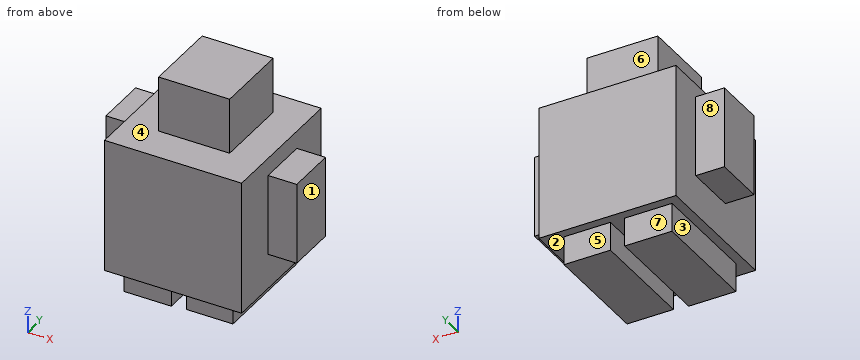
```python
from build123d import *

# Parameters (mm, degrees)
F0_W      = 74.0942507982
F0_H      = 74.6015533805
F1_DEPTH  = 72.4732205272
F2_W      = 38.3877456188
F2_H      = 40.8380180597
F3_DEPTH  = 30.0961155444
F4_W      = 26.9601941109
F4_H      = 43.9190119505
F5_DEPTH  = 15.5
F6_W      = 27.8298556805
F6_H      = 43.9190119505
F7_DEPTH  = 15.5
F8_W      = 25.5186259747
F8_H      = 59.9911510944
F9_DEPTH  = 15.5
F10_W     = 25.0709354877
F10_H     = 59.0957701206
F11_DEPTH = 15.5


with BuildPart() as f1:
    # F0 (on Top) → F1 (new body)
    with BuildSketch(Plane.XY):
        with Locations((-37.0471253991, 37.3007766902)):
            Rectangle(F0_W, F0_H)
    extrude(amount=F1_DEPTH)

    # F2 (on face) → F3 (join)
    with BuildSketch(Plane.XY.offset(72.4732205272)):
        with Locations((-36.9584262371, 40.0212556124)):
            Rectangle(F2_W, F2_H)
    extrude(amount=F3_DEPTH)

    # F4 (on face) → F5 (join)
    with BuildSketch(Plane.YZ):
        with Locations((38.2660329342, 40.9622490406)):
            Rectangle(F4_W, F4_H)
    extrude(amount=F5_DEPTH)

    # F6 (on face) → F7 (join)
    with BuildSketch(Plane(origin=(-74.0942507982, 0, 0), x_dir=(0, -1, 0), z_dir=(-1, 0, 0))):
        with Locations((-42.1796441078, 43.3538928628)):
            Rectangle(F6_W, F6_H)
    extrude(amount=F7_DEPTH)

    # F8 (on face) → F9 (join)
    with BuildSketch(Plane(origin=(0, 0, 0), x_dir=(1, 0, 0), z_dir=(0, 0, -1))):
        with Locations((-56.3197880983, -39.6210104227)):
            Rectangle(F8_W, F8_H)
    extrude(amount=F9_DEPTH)

    # F10 (on face) → F11 (join)
    with BuildSketch(Plane(origin=(0, 0, 0), x_dir=(1, 0, 0), z_dir=(0, 0, -1))):
        with Locations((-23.4141945839, -40.2925610542)):
            Rectangle(F10_W, F10_H)
    extrude(amount=F11_DEPTH)


solid = f1.part
```
The model under review builds one solid part; all positions refer to its coordinate system, in mm. Face numbers are marked on the shaded views. A direction names the side the tool comes from. Round coordinates to 2 decimals unless told otherwise and drop trailing zeros. Write each loop counter-clockwise with the first axis right and the second up, starting at its lowest first coordinate (ties: lowest second). Pieces come first, ordered by that corner, then holes. Notation, with made-up numbers: (85.25, 40.25) - (128.25, 40.25) arc R18 cw to (128.25, 56.25) - close; hole circle Ø5 at (-28, 44.25). An arc over 180 degrees is marked (long way). Answer as CSV lines item,"result". Start each with the question number.
(1) We need section D-D on x = -48. State the section outline as (y, z) points.
(2) Draft analysis for pull direction X (two halves, no side actions). For the marked faces 1, 2, 3 and 4, state which applies: pulls with the +X half, pulls with the -X half, needs draft (parallel to the pull), parting line crosses it, or undercut.
(3) To check wall thickness, follow line 1 (Y direction, x = -20.5, z = 96.5); line 2 (X direction, y = 60, z = 34.5); line 3 (Y direction, x = -77.5, z = 57). State the ranges of each line that lie inside material, in increasing order.
(4) We need section C-C on z = 61. State the section outline as (x, y) points.
(5) For the marked faces 5, 6, 7 and 8, list the 3-axis set-ups (+Z, -Z, +X, -X, +Y, -Y) from which the entire face can be reached by the end or side of a thin tool; tool diameter is ignored.
(6) We need section A-A on y = 42. State the section outline as (x, z) points.
(7) We need section B-B on x = -62.5. State the section outline as (y, z) points, plus the area to 3 significant figures.
(8) For pin 1 Ø12.5 at (x, z) = (-51.5, -4) entering from +Y; pin 2 Ø8 at (x, z) = (-84, 37) entering from -Y; pin 3 Ø8 at (x, y) = (-85.5, 47) entering from +Z; pin 4 Ø4.5 at (y, z) = (32, -10) entering from +X, all flat-tipped, find the tip position at first contact; note any pin that passes through.
Worked answers:
1,outline,"(0, 0) - (9.63, 0) - (9.63, -15.5) - (69.62, -15.5) - (69.62, 0) - (74.6, 0) - (74.6, 72.47) - (60.44, 72.47) - (60.44, 102.57) - (19.6, 102.57) - (19.6, 72.47) - (0, 72.47) - close"
2,face 1,"pulls with the +X half"
2,face 2,"undercut"
2,face 3,"pulls with the -X half"
2,face 4,"needs draft"
3,line 1,"19.6 to 60.44"
3,line 2,"-74.09 to 0"
3,line 3,"28.26 to 56.09"
4,outline,"(-89.59, 28.26) - (-74.09, 28.26) - (-74.09, 0) - (0, 0) - (0, 24.79) - (15.5, 24.79) - (15.5, 51.75) - (0, 51.75) - (0, 74.6) - (-74.09, 74.6) - (-74.09, 56.09) - (-89.59, 56.09) - close"
5,face 5,"-Z, +X, -X, +Y"
5,face 6,"+Z, +X, -X, +Y"
5,face 7,"-Z, -X, +Y"
5,face 8,"+Z, -Z, -X, +Y"
6,outline,"(-89.59, 21.39) - (-74.09, 21.39) - (-74.09, 0) - (-69.08, 0) - (-69.08, -15.5) - (-43.56, -15.5) - (-43.56, 0) - (-35.95, 0) - (-35.95, -15.5) - (-10.88, -15.5) - (-10.88, 0) - (0, 0) - (0, 19) - (15.5, 19) - (15.5, 62.92) - (0, 62.92) - (0, 72.47) - (-17.76, 72.47) - (-17.76, 102.57) - (-56.15, 102.57) - (-56.15, 72.47) - (-74.09, 72.47) - (-74.09, 65.31) - (-89.59, 65.31) - close"
7,outline,"(0, 0) - (9.63, 0) - (9.63, -15.5) - (69.62, -15.5) - (69.62, 0) - (74.6, 0) - (74.6, 72.47) - (0, 72.47) - close"
7,area,"6,340 mm²"
8,pin 1,"y = 74.6"
8,pin 2,"y = 28.26"
8,pin 3,"z = 65.31"
8,pin 4,"x = -10.88"
